from build123d import *

# Parameters (mm, degrees)
BOSS_EXTRUDE1_DEPTH = 14
SKETCH2_W           = 18
SKETCH2_H           = 18
CUT_EXTRUDE1_DEPTH  = 21
SKETCH3_R           = 1.3
BOSS_EXTRUDE2_DEPTH = 1.5


with BuildPart() as part:
    # Sketch1 → Boss-Extrude1 (new, symmetric)
    with BuildSketch(Plane(origin=(0, 0, 0), x_dir=(0, 0, -1), z_dir=(1, 0, 0))):
        Polygon((-22.5, 0), (-22.5, 21), (22.5, 21), (22.5, 0), (20.375, 0), (20.375, 6), (12.125, 6), (12.125, 0), (-12.125, 0), (-12.125, 6), (-20.375, 6), (-20.375, 0), align=None)
        Polygon((0, 10.900813089), (3.55, 12.950406544), (3.55, 17.049593456), (0, 19.099186911), (-3.55, 17.049593456), (-3.55, 12.950406544), align=None, mode=Mode.SUBTRACT)
    extrude(amount=BOSS_EXTRUDE1_DEPTH, both=True)

    # Sketch2 → Cut-Extrude1 (cut)
    with BuildSketch(Plane(origin=(0, 21, 0), x_dir=(1, 0, 0), z_dir=(0, 1, 0))):
        with Locations((-14, 0)):
            Rectangle(SKETCH2_W, SKETCH2_H)
        with Locations((14, 0)):
            Rectangle(SKETCH2_W, SKETCH2_H)
    extrude(amount=-CUT_EXTRUDE1_DEPTH, mode=Mode.SUBTRACT)

    # Sketch3 → Boss-Extrude2 (add)
    with BuildSketch(Plane(origin=(0, 21, 0), x_dir=(1, 0, 0), z_dir=(0, 1, 0))):
        Polygon((-5, -9), (-5, 9), (-14, 22.5), (-45, 9), (-45, -9), (-14, -22.5), align=None)
        with Locations(Location((-40, 4.5, 0), (0, 0, 270))):
            Circle(SKETCH3_R, mode=Mode.SUBTRACT)
        with Locations(Location((-40, -4.5, 0), (0, 0, 90))):
            Circle(SKETCH3_R, mode=Mode.SUBTRACT)
    extrude(amount=-BOSS_EXTRUDE2_DEPTH)


solid = part.part
Check sheet for the modelled part. Datum: model origin and axes. Units: mm. A direction names the side the tool comes from. Give positions to 0.01 mm unless a question says otherwise; leave off trailing zeros. Write each loop counter-clockwise with the first axis right and the second up, starting at its lowest first coordinate (ties: lowest second). Pieces come first, ordered by that corner, then holes. Notation, with made-up numbers: (15.5, 9.5) -> (50.5, 9.5) arc R28 cw to (50.5, 44.5) -> close; hole circle Ø10 at (-31, 47). An arc over 180 degrees is marked (long way). One line per item, written item: value. Start each with the question number.
Item 1: Section check A-A on z = -4.5. Record the cut outline in (x, y).
Item 2: Section check B-B on x = 9. Record the cut outline in (y, z) (3 decimals), then the cut area to 3 significant figures.
Item 3: Draft check along Y on faces 5 (the flat face through (0, 15, -3.55)), 6 (the flat face through (0, 0, -21)), 7 (the cylindrical face through (-38.71, 20.26, -4.67)). Enter one of: +Y half, -Y half, draft (parallel to the pull), parting line (faces both ways), or undercut.
Item 4: Tool access check on faces 1 (the flat face through (0.07, 11.94, 1.8)), 2 (the flat face through (-5, 10, 0)), 3 (the flat face through (-14, 12, 16)), 4 (the flat face through (5, 10.6, 0.1)). Record the directions out of +Z, -Z, +X, -X, +Y, -Y that give a thin tool (end or side, any length) a straight path to the whole face; none if there is none.
Item 5: Material ranges on probe 1 along Z at (x, y) = (-3.5, 14.25); probe 2 along X at (y, z) = (20.5, -4.5); probe 3 along X at (y, z) = (12.75, -6.5), recorded low to high. Write a range as from..to.
Item 6: Section check D-D on y = 1.75. Record the cut outline in (x, z) (3 decimals), then the cut area to 3 significant figures.
Item 7: Gauge pin test, flat ends, axial feed: pin 1 (11 mm diameter, centred on y = 5.5, z = -13.5, fed in from -X); pin 2 (8 mm diameter, centred on x = -21.5, z = -5.5, fed in from -Y); pin 3 (5 mm diameter, centred on y = 9, z = 0, fed in from -X). Record the tip position at first contact, or that the pin passes through.
Item 8: Section check C-C on y = 15. Record the cut outline in (x, z).
Results list:
1. outline: (-45, 19.5) -> (-41.3, 19.5) -> (-41.3, 21) -> (-45, 21) -> close; (-38.7, 19.5) -> (-5, 19.5) -> (-5, 0) -> (5, 0) -> (5, 21) -> (-38.7, 21) -> close
2. outline: (0, -22.5) -> (21, -22.5) -> (21, -9) -> (0, -9) -> (0, -12.125) -> (6, -12.125) -> (6, -20.375) -> (0, -20.375) -> close; (0, 9) -> (21, 9) -> (21, 22.5) -> (0, 22.5) -> (0, 20.375) -> (6, 20.375) -> (6, 12.125) -> (0, 12.125) -> close
2. area: 468 mm²
3. face 5: undercut
3. face 6: -Y half
3. face 7: draft
4. face 1: +X, -X
4. face 2: -X, -Y
4. face 3: +Z, -Z, -X, -Y
4. face 4: +X, +Y, -Y
5. probe 1: -22.5..-3.55, 3.55..22.5
5. probe 2: -45..-41.3, -38.7..5
5. probe 3: -5..5
6. outline: (-14, -22.5) -> (14, -22.5) -> (14, -20.375) -> (-14, -20.375) -> close; (-14, -12.125) -> (14, -12.125) -> (14, -9) -> (5, -9) -> (5, 9) -> (14, 9) -> (14, 12.125) -> (-14, 12.125) -> (-14, 9) -> (-5, 9) -> (-5, -9) -> (-14, -9) -> close; (-14, 20.375) -> (14, 20.375) -> (14, 22.5) -> (-14, 22.5) -> close
6. area: 474 mm²
7. pin 1: x = -14
7. pin 2: y = 19.5
7. pin 3: x = -5
8. outline: (-14, -22.5) -> (14, -22.5) -> (14, -9) -> (5, -9) -> (5, -3.55) -> (-5, -3.55) -> (-5, -9) -> (-14, -9) -> close; (-14, 9) -> (-5, 9) -> (-5, 3.55) -> (5, 3.55) -> (5, 9) -> (14, 9) -> (14, 22.5) -> (-14, 22.5) -> close
